The listing builds one solid part. Answer for the finished solid, in the listing's coordinates (mm). A direction names the side the tool comes from. Give positions to 0.01 mm unless a question says otherwise; leave off trailing zeros. Order: outer loops, then holes, each group sorted by start corner. A loop starts at its lowest first (then second) coordinate and runs counter-clockwise, first axis right, second up.
```python
from build123d import *

# Parameters (mm, degrees)
SKETCH014_W  = 9.5
SKETCH014_H  = 9.85
PAD007_DEPTH = 0.3
SKETCH015_W  = 0.3
SKETCH015_H  = 3
PAD008_DEPTH = 2.2
SKETCH016_W  = 0.3
SKETCH016_H  = 1
PAD009_DEPTH = 3.5


with BuildPart() as part:
    # Sketch014 → Pad007 (new body)
    with BuildSketch(Plane.XY):
        with Locations((0, -0.075)):
            Rectangle(SKETCH014_W, SKETCH014_H)
    extrude(amount=-PAD007_DEPTH)

    # Sketch015 → Pad008 (join)
    with BuildSketch(Plane.XY.offset(-0.3)):
        with Locations((-4.6, 0)):
            Rectangle(SKETCH015_W, SKETCH015_H)
    extrude(amount=-PAD008_DEPTH)

    # Sketch016 → Pad009 (join)
    with BuildSketch(Plane.XY.offset(-2.5)):
        with Locations((-4.6, 0)):
            Rectangle(SKETCH016_W, SKETCH016_H)
    extrude(amount=-PAD009_DEPTH)


solid = part.part
```
1) A tool of negligible diameter and unlimited length cuts with its end or side. For faces 1 (the flat face through (-4.45, 0, -2)), 2 (the flat face through (0, 0, 0)), from which of +Z, -Z, +X, -X, +Y, -Y can it reach the whole face along a straight path? Write none if from no direction.
Geometry says:
face 1: -Z, +X, +Y, -Y
face 2: +Z, +X, -X, +Y, -Y
2) Find section B-B (z = -0.95). Write down the section's boundary in (x, y).
Geometry says:
outline: (-4.75, -1.5) - (-4.45, -1.5) - (-4.45, 1.5) - (-4.75, 1.5) - close
3) Given P1, Ø5, axis at x = -3, y = -3.5, coming from the +Z side; P2, Ø2.5, axis at y = 0, z = -4.5, coming from the +X side; P3, Ø5, axis at x = 0.5, y = 3, coming from the -Z side, each flat-ended and moving along its own axis, determine where each tip first touches the part or whether it passes through.
Geometry says:
P1: stops at z = 0
P2: stops at x = -4.45
P3: stops at z = -0.3
4) Find section D-D (y = -0.75). Write down the section's boundary in (x, z), then the cut area to 3 significant figures.
Geometry says:
outline: (-4.75, -2.5) - (-4.45, -2.5) - (-4.45, -0.3) - (4.75, -0.3) - (4.75, 0) - (-4.75, 0) - close
area: 3.51 mm2
5) Find section C-C (x = 0.25). Write down the section's boundary in (y, z).
Geometry says:
outline: (-5, -0.3) - (4.85, -0.3) - (4.85, 0) - (-5, 0) - close
6) Find section A-A (y = 0.25). Write down the section's boundary in (x, z), then the cut area to 3 significant figures.
Geometry says:
outline: (-4.75, -6) - (-4.45, -6) - (-4.45, -0.3) - (4.75, -0.3) - (4.75, 0) - (-4.75, 0) - close
area: 4.56 mm2
7) Straight lines are drawn through the part: probe 1 along Z at (x, y) = (2.75, -0.5); probe 2 along X at (y, z) = (-0.25, -3.15). For each, find the intervals that lie inside material, in ascending order.
Geometry says:
probe 1: z = -0.3 to 0
probe 2: x = -4.75 to -4.45
